Geometry: final body of the model. Coordinates: model frame, mm. A direction names the side the tool comes from. Give positions to 0.01 mm unless a question says otherwise; leave off trailing zeros. Loops run counter-clockwise (first coordinate to the right, second up) from the corner with the lowest first, then second, coordinate; pieces in that order, holes last. Notation, with made-up numbers: (76.25, 72) - (83.25, 72) arc R15 cw to (83.25, 93) - close; hole circle Ø9 at (-22, 79.25). An arc over 180 degrees is marked (long way). Use one line per item in the form item = value.
```python
from build123d import *

# Parameters (mm, degrees)
F0_R     = 7.5
F1_DEPTH = 4
F2_R     = 5
F3_DEPTH = 54
F4_R     = 4
F5_DEPTH = 46


with BuildPart() as f1:
    # F0 (on Top) → F1 (new body)
    with BuildSketch(Plane.XY):
        Circle(F0_R)
    extrude(amount=F1_DEPTH)

    # F2 (on Top) → F3 (join)
    with BuildSketch(Plane.XY):
        Circle(F2_R)
    extrude(amount=F3_DEPTH)

    # F4 (on face) → F5 (join)
    with BuildSketch(Plane.XY.offset(54)):
        Circle(F4_R)
    extrude(amount=F5_DEPTH)


solid = f1.part
```
(1) Cut plane D-D (y = 6). Return the cut outline in (x, z).
Solution:
outline = (-4.5, 0) - (4.5, 0) - (4.5, 4) - (-4.5, 4) - close
(2) Pin query (flat end, axial travel): P1, Ø6, axis at x = -2, z = 54, coming from the -Y side; P2, Ø3, axis at y = -2.5, z = 65, coming from the +X side; P3, Ø6, axis at x = -3.5, z = 14.5, coming from the +Y side; P4, Ø5, axis at x = 5, y = 2, coming from the +Z side. Return the tip coordinate at first contact, or that it passes through.
Solution:
P1 = -5
P2 = 3.87
P3 = 4.97
P4 = 100
(3) Cut plane A-A (y = 0). Return the cut outline in (x, z).
Solution:
outline = (-7.5, 0) - (7.5, 0) - (7.5, 4) - (5, 4) - (5, 54) - (4, 54) - (4, 100) - (-4, 100) - (-4, 54) - (-5, 54) - (-5, 4) - (-7.5, 4) - close
(4) Access query for faces 1 (the face through (-1.08, -4.88, 28.65)), 2 (the face through (-7.493, 0.33, 1.972)). Directions: +Z, -Z, +X, -X, +Y, -Y. A direction counts if a zero-diameter tool reaches every point of the face in a straight line with its end or side. Return the directions, or none.
Solution:
face_1 = +Z
face_2 = +Z, -Z
(5) Cut plane C-C (z = 59). Return the cut outline in (x, y), plus the area to 3 significant figures.
Solution:
outline = circle Ø8 at (0, 0)
area = 50.3 mm2
(6) Material intervals for L1, parallel to Z at x = -6.25, y = 4; L2, parallel to Z at x = -3.25, y = -2.75; L3, parallel to Y at x = 0, z = 67.5, sorted ascending. Write a range as from..to.
Solution:
L1 = 0..4
L2 = 0..54
L3 = -4..4
